from build123d import *

# Parameters (mm, degrees)
SCHIZZO1_W                   = 36
SCHIZZO1_H                   = 22
ESTRUSIONE_ESTRUSIONE1_DEPTH = 18
RACCORDO1_R                  = 3
ESTRUSIONE_ESTRUSIONE2_DEPTH = 28
SCHIZZO3_R                   = 2.5
ESTRUSIONE_ESTRUSIONE3_DEPTH = 8
SCHIZZO3_4_R                 = 1.5
TAGLIO_ESTRUSIONE1_DEPTH     = 19


with BuildPart() as part:
    # Schizzo1 → Estrusione-Estrusione1 (new body)
    with BuildSketch(Plane.XY):
        Rectangle(SCHIZZO1_W, SCHIZZO1_H)
    extrude(amount=ESTRUSIONE_ESTRUSIONE1_DEPTH)

    # Raccordo1
    raccordo1_edges = [part.edges().sort_by_distance(p)[0] for p in [
        (18, 11, 9),
        (18, -11, 9),
    ]]
    fillet(raccordo1_edges, radius=RACCORDO1_R)

    # Schizzo2 → Estrusione-Estrusione2 (add)
    with BuildSketch(Plane.ZY.offset(18)):
        with BuildLine():
            Line((1.5, 7), (1.5, -7))
            ThreePointArc((1.5, -7), (9.883293707, -10.640228974), (18, -6.439043509))
            Line((18, -6.439043509), (18, 6.439043509))
            ThreePointArc((18, 6.439043509), (9.883293707, 10.640228974), (1.5, 7))
        make_face()
    extrude(amount=ESTRUSIONE_ESTRUSIONE2_DEPTH)

    # Schizzo3 → Estrusione-Estrusione3 (add)
    with BuildSketch(Plane(origin=(0, 0, 0), x_dir=(-1, 0, 0), z_dir=(0, 0, -1))):
        with Locations((-6, 0)):
            Circle(SCHIZZO3_R)
    extrude(amount=ESTRUSIONE_ESTRUSIONE3_DEPTH)

    # Schizzo3<4> → Taglio-Estrusione1 (cut, through all)
    with BuildSketch(Plane(origin=(0, 0, 0), x_dir=(-1, 0, 0), z_dir=(0, 0, -1))):
        with Locations((13, 8.5)):
            Circle(SCHIZZO3_4_R)
        with Locations((13, -8.5)):
            Circle(SCHIZZO3_4_R)
    extrude(amount=-TAGLIO_ESTRUSIONE1_DEPTH, mode=Mode.SUBTRACT)


solid = part.part
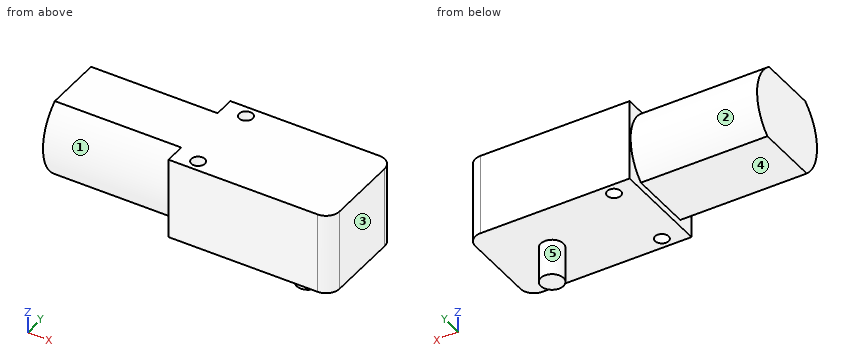
The model under review builds one solid part; all positions refer to its coordinate system, in mm. Face numbers are marked on the shaded views. A direction names the side the tool comes from. Coordinates: 2 decimals unless noted, no trailing zeros. Loops run counter-clockwise (first coordinate to the right, second up) from the corner with the lowest first, then second, coordinate; pieces in that order, holes last.
(1) Insertion check: P1, Ø1.5, axis at y = 3.5, z = -1.5, coming from the +X side; P2, Ø3, axis at x = -36, z = 5.5, coming from the -Y side; P3, Ø7, axis at x = -33.5, y = 0.5, coming from the -Z side; P4, Ø1, axis at x = -6.5, y = -3, coming from the -Z side. Each pin has a flat end and moves straight along its axis. Give the tip position at first contact, or say it passes through.
Determined:
P1: passes through
P2: stops at y = -10.34
P3: stops at z = 1.5
P4: stops at z = 0
(2) Consider section B-B, the plane y = 0. Give the boundary of the cut face in (x, z).
Determined:
outline: (-46, 1.5) - (-18, 1.5) - (-18, 0) - (3.5, 0) - (3.5, -8) - (8.5, -8) - (8.5, 0) - (18, 0) - (18, 18) - (-46, 18) - close
(3) Consider section D-D, the plane z = -4.25. Give the boundary of the cut face in (x, y), plus the area to 3 significant figures.
Determined:
outline: circle Ø5 at (6, 0)
area: 19.6 mm2
(4) Consider section A-A, the plane x = -13. Give the boundary of the cut face in (y, z).
Determined:
outline: (-11, 0) - (-10, 0) - (-10, 18) - (-11, 18) - close; (-7, 0) - (7, 0) - (7, 18) - (-7, 18) - close; (10, 0) - (11, 0) - (11, 18) - (10, 18) - close
(5) Tool access review of the marked faces 1, 2, 3, 4 and 5: name each direction out of +Z, -Z, +X, -X, +Y, -Y from which nothing blocks a thin tool from reaching the whole face with its end or side.
Determined:
face 1: -X, -Y
face 2: -X, +Y
face 3: +Z, -Z, +X, +Y, -Y
face 4: -Z, -X, +Y, -Y
face 5: -Z
(6) Wall thickness on L1, parallel to Y at x = -13, z = 8.75; L2, parallel to Z at x = -2, y = 4.5; L3, parallel to Z at x = -37, y = 2.75: over which ranges is each line inside the solid? List them lowest first.
Determined:
L1: y = -11 to -10, -7 to 7, 10 to 11
L2: z = 0 to 18
L3: z = 1.5 to 18
(7) Consider section C-C, the plane z = 16. Give the boundary of the cut face in (x, y), plus the area to 3 significant figures.
Determined:
outline: (-46, -8.45) - (-18, -8.45) - (-18, -11) - (15, -11) arc R3 ccw to (18, -8) - (18, 8) arc R3 ccw to (15, 11) - (-18, 11) - (-18, 8.45) - (-46, 8.45) - close; hole circle Ø3 at (-13, -8.5); hole circle Ø3 at (-13, 8.5)
area: 1,250 mm2
